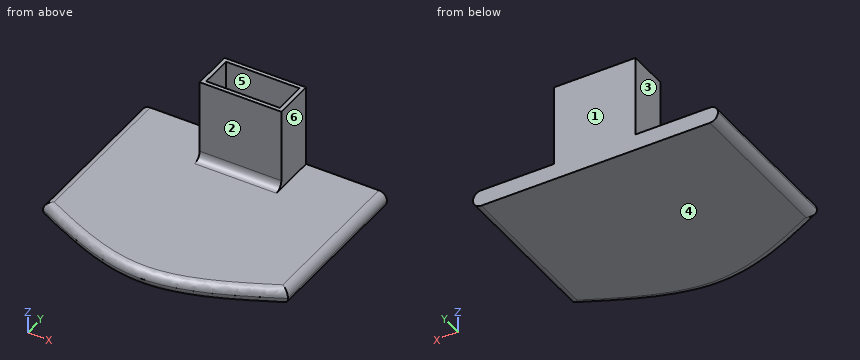
```python
from build123d import *

# Parameters (mm, degrees)
F1_DEPTH = 10
F2_W     = 50
F2_H     = 25
F3_DEPTH = 50
F4_T     = -2.5
F5_R     = 4.999


# Not quite as in the source:
# - a fillet or chamfer is up to 0.001 mm smaller than in the source, because OpenCascade refuses the exact size


with BuildPart() as f1:
    # F0 (on Top) → F1 (new body)
    with BuildSketch(Plane.XY):
        with BuildLine():
            Line((75, 50), (-75, 50))
            Line((-75, 50), (-75, -50))
            add(Edge.make_bspline(
                [(-75, -50), (-50, -62.5487543643), (0, -87.6462630928), (50, -62.5487543643), (75, -50)],
                knots=[0, 0, 0, 0, 0.5, 1, 1, 1, 1], degree=3))
            Line((75, -50), (75, 50))
        make_face()
    extrude(amount=F1_DEPTH)

    # F2 (on face) → F3 (join)
    with BuildSketch(Plane.XY.offset(10)):
        with Locations((0.4496160895, 37.5)):
            Rectangle(F2_W, F2_H)
    extrude(amount=F3_DEPTH)

    # F4
    f4_openings = [f1.faces().sort_by_distance(p)[0] for p in [
        (0.449616, 37.5, 60),
    ]]
    offset(amount=F4_T, openings=f4_openings, kind=Kind.INTERSECTION)

    # F5 (radius 5 in the source; OpenCascade refuses exactly that, so slightly less here)
    f5_edges = [f1.edges().sort_by_distance(p)[0] for p in [
        (0, -75.097509, 10),
        (0, -75.097509, 0),
        (-75, 0, 10),
        (-75, 0, 0),
        (75, 0, 0),
        (75, 0, 10),
        (0.449616, 25, 10),
    ]]
    fillet(f5_edges, radius=F5_R)


solid = f1.part
```
The model under review builds one solid part; all positions refer to its coordinate system, in mm. Face numbers are marked on the shaded views. A direction names the side the tool comes from. Round coordinates to 2 decimals unless told otherwise and drop trailing zeros. Loops run counter-clockwise (first coordinate to the right, second up) from the corner with the lowest first, then second, coordinate; pieces in that order, holes last. Notation, with made-up numbers: M -1,11.25 L 45,11.25 A22 ccw 45,47.25 Z; hole C 27.5,36 d4. An arc over 180 degrees is marked long. Put each result on its own line as item: value.
Q1. Consider section A-A, the plane z = 42.5. Give the boundary of the cut face in (x, y).
Result set:
outline: M -24.55,25 L 25.45,25 L 25.45,50 L -24.55,50 Z; hole M -22.05,27.5 L 22.95,27.5 L 22.95,47.5 L -22.05,47.5 Z
Q2. Machinability: for the marked faces 1, 2 and 3, which of the approach directions +Z, -Z, +X, -X, +Y, -Y give a long, thin tool a straight path to every point of the face, cutting with its end or side? Answer none if there is none.
Result set:
face 1: +Z, -Z, +X, -X, +Y
face 2: +Z, +X, -X, -Y
face 3: +Z, -X, +Y, -Y
Q3. To check wall thickness, follow L1, parallel to Z at x = -1, y = -15.5; L2, parallel to Y at x = -7, z = 38; L3, parallel to Z at x = -23.5, y = 43.5. State the ranges of each line that lie inside material, in increasing order.
Result set:
L1: z = 0 to 2.5, 7.5 to 10
L2: y = 25 to 27.5, 47.5 to 50
L3: z = 0 to 2.5, 7.5 to 60
Q4. Mouldability with a two-part tool opening along X and no side actions: class the marked faces 4, 5 and 6 as released by +X, released by -X, zero draft, split by the parting line, or undercut.
Result set:
face 4: zero draft
face 5: undercut
face 6: released by +X
Q5. For pin 1 (9 mm diameter, centred on y = 31, z = 36.5, fed in from -X); pin 2 (1.5 mm diameter, centred on y = -18.5, z = 4, fed in from -X); pin 3 (6 mm diameter, centred on y = 32.5, z = 10.5, fed in from +X), all flat-tipped, find the tip position at first contact; note any pin that passes through.
Result set:
pin 1: stops at x = -24.55
pin 2: stops at x = -74.99
pin 3: stops at x = 74.33
